Read the model definition and answer for the solid it produces. Units are mm, in the model's axes. A direction names the side the tool comes from. Coordinates: 2 decimals unless noted, no trailing zeros. Loops run counter-clockwise (first coordinate to the right, second up) from the corner with the lowest first, then second, coordinate; pieces in that order, holes last.
from build123d import *

# Parameters (mm, degrees)
BOSS_EXTRUDE1_DEPTH = 3.2
SKETCH2_W           = 159.499713068
SKETCH2_H           = 43.7032655
CUT_EXTRUDE1_DEPTH  = 3.2
FILLET1_R           = 0.5


with BuildPart() as part:
    # Sketch1 → Boss-Extrude1 (new body)
    with BuildSketch(Plane(origin=(0, 0, 0), x_dir=(1, 0, 0), z_dir=(0, 1, 0))):
        with BuildLine():
            Line((-52.508964924, -8.867320879), (-52.508964924, -23.867320879))
            Line((-52.508964924, -23.867320879), (90.983964924, -23.867320879))
            Line((90.983964924, -23.867320879), (90.983964924, -3.232453337))
            ThreePointArc((90.983964924, -3.232453337), (84.775, -7), (78.566035076, -3.232453337))
            ThreePointArc((78.566035076, -3.232453337), (73.2, -1.808851774), (67.833964924, -3.232453337))
            ThreePointArc((67.833964924, -3.232453337), (61.625, -7), (55.416035076, -3.232453337))
            ThreePointArc((55.416035076, -3.232453337), (50.05, -1.808851774), (44.683964924, -3.232453337))
            ThreePointArc((44.683964924, -3.232453337), (38.475, -7), (32.266035076, -3.232453337))
            Line((32.266035076, -3.232453337), (21.492035076, -3.232453337))
            Line((21.492035076, -3.232453337), (6.208964923, -8.867320879))
            ThreePointArc((6.208964923, -8.867320879), (0, -10.825), (-6.208964924, -8.867320879))
            ThreePointArc((-6.208964924, -8.867320879), (-11.575, -6.362392354), (-16.941035077, -8.867320879))
            ThreePointArc((-16.941035077, -8.867320879), (-23.15, -10.825), (-29.358964924, -8.867320879))
            ThreePointArc((-29.358964924, -8.867320879), (-34.725, -6.362392354), (-40.091035076, -8.867320879))
            ThreePointArc((-40.091035076, -8.867320879), (-46.3, -10.825), (-52.508964924, -8.867320879))
        make_face()
    extrude(amount=BOSS_EXTRUDE1_DEPTH)

    # Sketch2 → Cut-Extrude1 (cut)
    with BuildSketch(Plane(origin=(0, 3.2, 0), x_dir=(1, 0, 0), z_dir=(0, 1, 0))):
        with Locations((19.511770452, -6.74153154)):
            Rectangle(SKETCH2_W, SKETCH2_H)
        with BuildLine():
            Line((-52.008964924, -9.780764004), (-52.008964924, -23.367320879))
            Line((-52.008964924, -23.367320879), (90.483964924, -23.367320879))
            Line((90.483964924, -23.367320879), (90.483964924, -4.863920178))
            ThreePointArc((90.483964924, -4.863920178), (84.005832381, -7.460454488), (78.193740084, -3.596806627))
            ThreePointArc((78.193740084, -3.596806627), (73.2, -2.308851774), (68.206259916, -3.596806627))
            ThreePointArc((68.206259916, -3.596806627), (61.625, -7.5), (55.043740084, -3.596806627))
            ThreePointArc((55.043740084, -3.596806627), (50.05, -2.308851774), (45.056259916, -3.596806627))
            ThreePointArc((45.056259916, -3.596806627), (38.552735975, -7.49959713), (31.969710453, -3.732453337))
            Line((31.969710453, -3.732453337), (21.581273902, -3.732453337))
            Line((21.581273902, -3.732453337), (6.442002791, -9.314302177))
            ThreePointArc((6.442002791, -9.314302177), (-0.066748771, -11.324803292), (-6.551349026, -9.237718925))
            ThreePointArc((-6.551349026, -9.237718925), (-11.575, -6.862392354), (-16.598650974, -9.237718925))
            ThreePointArc((-16.598650974, -9.237718925), (-23.15, -11.325), (-29.701349026, -9.237718925))
            ThreePointArc((-29.701349026, -9.237718925), (-34.725, -6.862392354), (-39.748650974, -9.237718925))
            ThreePointArc((-39.748650974, -9.237718925), (-45.798874034, -11.313907272), (-52.008964924, -9.780764004))
        make_face(mode=Mode.SUBTRACT)
    extrude(amount=-CUT_EXTRUDE1_DEPTH, mode=Mode.SUBTRACT)

    # Fillet1
    fillet1_edges = [part.edges().sort_by_distance(p)[0] for p in [
        (21.581273902, 1.6, 3.732453337),
        (31.969710453, 1.6, 3.732453337),
        (90.483964924, 1.6, 4.863920178),
        (90.483964924, 1.6, 23.367320879),
        (-52.008964924, 1.6, 23.367320879),
        (-52.008964924, 1.6, 9.780764004),
    ]]
    fillet(fillet1_edges, radius=FILLET1_R)


solid = part.part
Item 1: Find the intervals of material crossed by line 1 along Z through (x, y) = (-23, 0.75); line 2 along Z through (x, y) = (68, 1.3), in increasing order.
Numbers:
line 1: z = 11.32 to 23.37
line 2: z = 3.95 to 23.37
Item 2: A cutting plane is placed at B-B on x = 0. Determine the outline of the cut face in (y, z) (3 decimals).
Numbers:
outline: (0, 11.325) - (3.2, 11.325) - (3.2, 23.367) - (0, 23.367) - close
Item 3: A cutting plane is placed at C-C on x = 63. Determine the outline of the cut face in (y, z).
Numbers:
outline: (0, 7.37) - (3.2, 7.37) - (3.2, 23.37) - (0, 23.37) - close
Item 4: Determine the mould class of faces 1 (the face through (-11.495, 1.622, 6.863)), 2 (the face through (-52.009, 2, 17)), 3 (the face through (18, 0, 15)) for opening direction X: released by +X, released by -X, zero draft, split by the parting line, or undercut.
Numbers:
face 1: undercut
face 2: released by -X
face 3: zero draft
Item 5: A cutting plane is placed at A-A on y = 2.05. Determine the outline of the cut face in (x, z) (3 decimals).
Numbers:
outline: (-52.009, 10.616) arc R0.5 ccw to (-51.289, 10.167) arc R11.325 cw to (-39.749, 9.238) arc R6.5 ccw to (-29.701, 9.238) arc R11.325 cw to (-16.599, 9.238) arc R6.5 ccw to (-6.551, 9.238) arc R11.325 cw to (6.442, 9.314) - (21.498, 3.763) arc R0.5 ccw to (21.671, 3.732) - (31.686, 3.732) arc R0.5 ccw to (32.111, 3.968) arc R7.5 cw to (45.056, 3.597) arc R10.325 ccw to (55.044, 3.597) arc R7.5 cw to (68.206, 3.597) arc R10.325 ccw to (78.194, 3.597) arc R7.5 cw to (89.658, 5.692) arc R0.5 ccw to (90.484, 6.072) - (90.484, 22.867) arc R0.5 ccw to (89.984, 23.367) - (-51.509, 23.367) arc R0.5 ccw to (-52.009, 22.867) - close
Item 6: Given pin 1 (1 mm diameter, centred on x = 57.5, y = 0.5, fed in from -Z); pin 2 (1.6 mm diameter, centred on x = 28.5, y = 1, fed in from -Z); pin 3 (6 mm diameter, centred on x = 37.5, z = 4.5, fed in from -Y), each flat-ended and moving along its own axis, determine where each tip first touches the part or whether it passes through.
Numbers:
pin 1: stops at z = 5.9
pin 2: stops at z = 3.73
pin 3: stops at y = 0
Item 7: Which of the six approach directions +Z, -Z, +X, -X, +Y, -Y give full straight-line access (tool end or side, diameter ignored) to faces 4 (the face through (27, 2, 3.732)), 5 (the face through (14.08, 1.62, 6.5)), 6 (the face through (90.484, 2, 15))?
Numbers:
face 4: -Z, -X, +Y, -Y
face 5: -Z, +Y, -Y
face 6: +Z, -Z, +X, +Y, -Y
